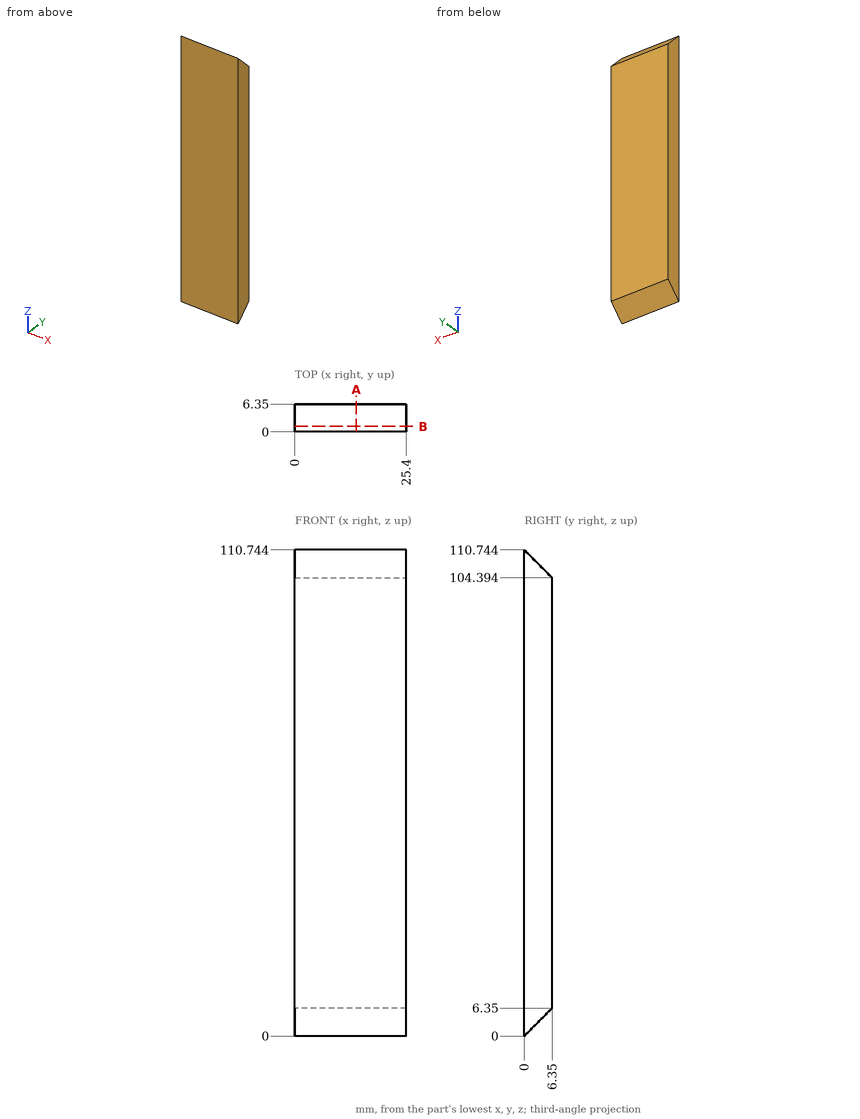
Design review of the part shown in the three views and the two pictorial views. Dimensions are in mm from the part's minimum x, y and z. Round coordinates to 2 decimals unless told otherwise and drop trailing zeros. Loops run counter-clockwise (first coordinate to the right, second up) from the corner with the lowest first, then second, coordinate; pieces in that order, holes last. Notation, with made-up numbers: (-39.75, -12.75) - (17.25, -12.75) arc R18 ccw to (17.25, -3.75) - close; hole circle Ø9 at (-18.75, -8.75). An arc over 180 degrees is marked (long way). Use CSV: the item, a comma, the result in double quotes.
(1) For line 1 (Z direction, x = 9.75, y = 5.75); line 2 (Z direction, x = 14, y = 4.5), list the stretches that pass through material, from the lowest coordinate up.
Working result:
line 1,"z = 5.75 to 104.99"
line 2,"z = 4.5 to 106.24"
(2) Take a section at B-B, the plane y = 1.25. Give the boundary of the cut face in (x, z), plus the area to 3 significant figures.
Working result:
outline,"(0, 1.25) - (25.4, 1.25) - (25.4, 109.49) - (0, 109.49) - close"
area,"2,750 mm^2"
(3) Clearance check with flat-ended pins moving along their axes: P1, Ø1.5, axis at x = 10.5, y = 1, coming from the +Z side; P2, Ø1, axis at x = 9, y = 5, coming from the +Z side. State where each tip first meets the part, or that it passes through.
Working result:
P1,"stops at z = 110.49"
P2,"stops at z = 106.24"
(4) Take a section at A-A, the plane x = 14. Give the boundary of the cut face in (y, z).
Working result:
outline,"(0, 0) - (6.35, 6.35) - (6.35, 104.39) - (0, 110.74) - close"
